Geometry check sheet. Reference: the model listing, model coordinates, mm. A direction names the side the tool comes from. Coordinates: 2 decimals unless noted, no trailing zeros. Loops run counter-clockwise (first coordinate to the right, second up) from the corner with the lowest first, then second, coordinate; pieces in that order, holes last. Notation, with made-up numbers: (76.5, 68) - (97.5, 68) arc R33 cw to (97.5, 104) - close; hole circle Ø8 at (-27, 68). An arc over 180 degrees is marked (long way). Write item = value, one per line. Start each with the question number.
from build123d import *

# Parameters (mm, degrees)
ESQUISSE1_R          = 25
ESQUISSE1_R_2        = 20
BOSS_EXTRU_3_DEPTH   = 1.5
ESQUISSE1_R_3        = 15
ESQUISSE1_R_4        = 10
BOSS_EXTRU_3_2_DEPTH = 1.5
ESQUISSE3_W          = 7
ESQUISSE3_H          = 3
ESQUISSE3_W_2        = 3
ESQUISSE3_H_2        = 7
BOSS_EXTRU_5_DEPTH   = 1.5


with BuildPart() as part:
    # Esquisse1 → Boss.-Extru.3 (new body)
    with BuildSketch(Plane(origin=(0, 0, 0), x_dir=(1, 0, 0), z_dir=(0, 1, 0))):
        Circle(ESQUISSE1_R)
        Circle(ESQUISSE1_R_2, mode=Mode.SUBTRACT)
    extrude(amount=BOSS_EXTRU_3_DEPTH)



with BuildPart() as body_2:
    # Esquisse1 → Boss.-Extru.3 2 (new body)
    with BuildSketch(Plane(origin=(0, 0, 0), x_dir=(1, 0, 0), z_dir=(0, 1, 0))):
        Circle(ESQUISSE1_R_3)
        Circle(ESQUISSE1_R_4, mode=Mode.SUBTRACT)
    extrude(amount=BOSS_EXTRU_3_2_DEPTH)


with BuildPart() as part_1:
    add(part.part)

    add(body_2.part)  # Boss.-Extru.5 merges body 2
    # Esquisse3 → Boss.-Extru.5 (add)
    with BuildSketch(Plane(origin=(0, 1.5, 0), x_dir=(-1, 0, 0), z_dir=(0, 1, 0))):
        with Locations((18.424811557, 0)):
            Rectangle(ESQUISSE3_W, ESQUISSE3_H)
        with Locations((0, -17.5)):
            Rectangle(ESQUISSE3_W_2, ESQUISSE3_H_2)
        with Locations((-17.5, 0)):
            Rectangle(ESQUISSE3_W, ESQUISSE3_H)
        with Locations((0, 17.5)):
            Rectangle(ESQUISSE3_W_2, ESQUISSE3_H_2)
    extrude(amount=-BOSS_EXTRU_5_DEPTH)


solid = part_1.part
(1) Scan lines: line 1 (Z direction, x = 0, y = 0.9); line 2 (X direction, y = 0.6, z = 18). Record each from-to range of solid material in increasing order.
(2) Sectioned sample at C-C on z = 0. Enter the section's corners in (x, y).
(3) Sectioned sample at A-A on x = 0. Enter the section's corners in (y, z).
(4) Sectioned sample at D-D on z = 14. Enter the section's corners in (x, y).
(5) Sectioned sample at B-B on y = 1.1. Enter the section's corners in (x, z), plus the area to 3 significant figures.
(6) Depth check by flat-ended pin: pin 1 (12 mm diameter, centred on x = 1.5, z = 5, fed in from -Y); pin 2 (0.8 mm diameter, centred on y = 0.5, z = -18.5, fed in from +X) (3 decimals); pin 3 (0.8 mm diameter, centred on y = 1, z = -17.5, fed in from -X); pin 4 (12 mm diameter, centred on x = 0, z = 0, fed in from +Y). Enter the tip coordinate at first touch or a pass-through.
(7) Draft check along Z on faces 3 (the face through (0, 1.5, 11)), 4 (the face through (-1.5, 1, 17)). Enter one of: pulls with the +Z half, pulls with the -Z half, needs draft (parallel to the pull), parting line crosses it, or undercut.
(8) Tool access check on faces 1 (the face through (0, 0, 11)), 2 (the face through (-17, 1, -1.5)). Record the directions out of +Z, -Z, +X, -X, +Y, -Y that give a thin tool (end or side, any length) a straight path to the whole face; none if there is none.
Working result:
q1.line_1 = -25 to -10, 10 to 25
q1.line_2 = -17.35 to -8.72, -1.5 to 1.5, 8.72 to 17.35
q2.outline = (-25, 0) - (-10, 0) - (-10, 1.5) - (-25, 1.5) - close; (10, 0) - (25, 0) - (25, 1.5) - (10, 1.5) - close
q3.outline = (0, -25) - (1.5, -25) - (1.5, -10) - (0, -10) - close; (0, 10) - (1.5, 10) - (1.5, 25) - (0, 25) - close
q4.outline = (-20.71, 0) - (-14.28, 0) - (-14.28, 1.5) - (-20.71, 1.5) - close; (-5.39, 0) - (5.39, 0) - (5.39, 1.5) - (-5.39, 1.5) - close; (14.28, 0) - (20.71, 0) - (20.71, 1.5) - (14.28, 1.5) - close
q5.outline = circle Ø50 at (0, 0); hole (-19.94, -1.5) arc R20 ccw to (-1.5, -19.94) - (-1.5, -14.92) arc R15 cw to (-14.92, -1.5) - close; hole (-19.94, 1.5) - (-14.92, 1.5) arc R15 cw to (-1.5, 14.92) - (-1.5, 19.94) arc R20 ccw to start; hole circle Ø20 at (0, 0); hole (1.5, -19.94) arc R20 ccw to (19.94, -1.5) - (14.92, -1.5) arc R15 cw to (1.5, -14.92) - close; hole (1.5, 14.92) arc R15 cw to (14.92, 1.5) - (19.94, 1.5) arc R20 ccw to (1.5, 19.94) - close
q5.area = 1,160 mm2
q6.pin_1 = 0
q6.pin_2 = 17.245
q6.pin_3 = -18.24
q6.pin_4 = through
q7.face_3 = needs draft
q7.face_4 = undercut
q8.face_1 = +Z, -Z, +X, -X, -Y
q8.face_2 = +Y, -Y
